Source: CAD feature listing. Evaluate the final solid. Frame: model axes, mm. A direction names the side the tool comes from. Coordinates: 2 decimals unless noted, no trailing zeros. Order: outer loops, then holes, each group sorted by start corner. A loop starts at its lowest first (then second) coordinate and runs counter-clockwise, first axis right, second up.
```python
from build123d import *

# Parameters (mm, degrees)
SKETCH_1_W          = 94
SKETCH_1_H          = 44
EXTRUDE_2_DEPTH     = 20
SKETCH_2_W          = 90
SKETCH_2_H          = 40
CUT_EXTRUDE_1_DEPTH = 19
SKETCH_3_W          = 5
SKETCH_3_H          = 5
EXTRUDE_3_DEPTH     = 35


with BuildPart() as part:
    # 草图1 → 凸台-拉伸2 (new body)
    with BuildSketch(Plane(origin=(0, 0, 0), x_dir=(1, 0, 0), z_dir=(0, 1, 0))):
        with Locations((47, 22)):
            Rectangle(SKETCH_1_W, SKETCH_1_H)
    extrude(amount=EXTRUDE_2_DEPTH)

    # 草图2 → 切除-拉伸1 (cut)
    with BuildSketch(Plane(origin=(0, 20, 0), x_dir=(1, 0, 0), z_dir=(0, 1, 0))):
        with Locations((47, 22)):
            Rectangle(SKETCH_2_W, SKETCH_2_H)
    extrude(amount=-CUT_EXTRUDE_1_DEPTH, mode=Mode.SUBTRACT)

    # 草图3 → 凸台-拉伸3 (add)
    with BuildSketch(Plane.XZ):
        with Locations((2.5, -2.5)):
            Rectangle(SKETCH_3_W, SKETCH_3_H)
        with Locations((91.5, -2.5)):
            Rectangle(SKETCH_3_W, SKETCH_3_H)
        with Locations((91.5, -41.5)):
            Rectangle(SKETCH_3_W, SKETCH_3_H)
        with Locations((2.5, -41.5)):
            Rectangle(SKETCH_3_W, SKETCH_3_H)
    extrude(amount=EXTRUDE_3_DEPTH)


solid = part.part
```
Q1. Section query C-C on y = 7. Output: boundary loops of the cut face in (x, z), plus the area to 3 significant figures.
Solutions:
outline: (0, -44) - (94, -44) - (94, 0) - (0, 0) - close; hole (2, -42) - (92, -42) - (92, -2) - (2, -2) - close
area: 536 mm2
Q2. Section query D-D on x = 8.5. Output: boundary loops of the cut face in (y, z), plus the area to 3 significant figures.
Solutions:
outline: (0, -44) - (20, -44) - (20, -42) - (1, -42) - (1, -2) - (20, -2) - (20, 0) - (0, 0) - close
area: 120 mm2
Q3. Pull-direction query (X, two-part tool) for faces 1 (the flat face through (92, 11, -22)), 2 (the flat face through (94, 4, -22)), 3 (the flat face through (2, -17, -39)); classes: pulls with the +X half, pulls with the -X half, needs draft (parallel to the pull), parting line crosses it, or undercut.
Solutions:
face 1: undercut
face 2: pulls with the +X half
face 3: needs draft
Q4. Section query A-A on y = -22. Output: boundary loops of the cut face in (x, z), plus the area to 3 significant figures.
Solutions:
outline: (0, -44) - (5, -44) - (5, -39) - (0, -39) - close; (0, -5) - (5, -5) - (5, 0) - (0, 0) - close; (89, -44) - (94, -44) - (94, -39) - (89, -39) - close; (89, -5) - (94, -5) - (94, 0) - (89, 0) - close
area: 100 mm2
Q5. Material intervals for line 1 along X through (y, z) = (-22.5, -1.5); line 2 along X through (y, z) = (15, -14); line 3 along Z through (x, y) = (82, 1.5), sorted ascending.
Solutions:
line 1: x = 0 to 5, 89 to 94
line 2: x = 0 to 2, 92 to 94
line 3: z = -44 to -42, -2 to 0
Q6. Pin query (flat end, axial travel): P1, Ø1, axis at x = 9.5, z = -13, coming from the -Y side; P2, Ø12, axis at x = 35.5, z = -22.5, coming from the +Y side. Return the tip coordinate at first contact, or that it passes through.
Solutions:
P1: stops at y = 0
P2: stops at y = 1
Q7. Set-up query: faces 4 (the flat face through (5, -17, -3)), 5 (the flat face through (46, 11, -42)), 6 (the flat face through (36, 5, 0)), 7 (the flat face through (2, -17, -5)). Return all of +Z, -Z, +X, -X, +Y, -Y with unobstructed straight access to the full face (end or side cutting, diameter ignored); none if empty.
Solutions:
face 4: +Z, -Z, -Y
face 5: +Y
face 6: +Z, +X, -X, +Y, -Y
face 7: +X, -X, -Y
Q8. Section query B-B on z = -20.5. Output: boundary loops of the cut face in (x, y).
Solutions:
outline: (0, 0) - (94, 0) - (94, 20) - (92, 20) - (92, 1) - (2, 1) - (2, 20) - (0, 20) - close
